Source: CAD feature listing. Evaluate the final solid. Frame: model axes, mm. A direction names the side the tool comes from. Round coordinates to 2 decimals unless told otherwise and drop trailing zeros. Write each loop counter-clockwise with the first axis right and the second up, starting at its lowest first coordinate (ties: lowest second). Pieces come first, ordered by that corner, then holes.
```python
from build123d import *

# Parameters (mm, degrees)
SKETCH1_R           = 2.54
BOSS_EXTRUDE1_DEPTH = 4.699
BOSS_EXTRUDE2_DEPTH = 50.419
FILLET1_R           = 3.81
FILLET2_R           = 2.54
FILLET3_R           = 1.27
SKETCH3_R           = 19.05
BOSS_EXTRUDE3_DEPTH = 1.524
CUT_EXTRUDE1_START  = -6.35
SKETCH5_R           = 22.225
CUT_EXTRUDE1_DEPTH  = 44.45
SKETCH4_R           = 3.175
BOSS_EXTRUDE4_DEPTH = 19.05


with BuildPart() as part:
    # Sketch1 → Boss-Extrude1 (new body)
    with BuildSketch(Plane(origin=(0, 0, 0), x_dir=(1, 0, 0), z_dir=(0, 1, 0))):
        with BuildLine():
            Line((-23.622, 28.575), (23.622, 28.575))
            ThreePointArc((23.622, 28.575), (27.124299887, 27.124299887), (28.575, 23.622))
            Line((28.575, 23.622), (28.575, -23.622))
            ThreePointArc((28.575, -23.622), (27.124299887, -27.124299887), (23.622, -28.575))
            Line((23.622, -28.575), (-23.622, -28.575))
            ThreePointArc((-23.622, -28.575), (-27.124299887, -27.124299887), (-28.575, -23.622))
            Line((-28.575, -23.622), (-28.575, 23.622))
            ThreePointArc((-28.575, 23.622), (-27.124299887, 27.124299887), (-23.622, 28.575))
        make_face()
        with Locations(Location((-23.622, 23.622, 0), (0, 0, 270))):
            Circle(SKETCH1_R, mode=Mode.SUBTRACT)
        with Locations(Location((23.622, 23.622, 0), (0, 0, 270))):
            Circle(SKETCH1_R, mode=Mode.SUBTRACT)
        with Locations(Location((23.622, -23.622, 0), (0, 0, 270))):
            Circle(SKETCH1_R, mode=Mode.SUBTRACT)
        with Locations(Location((-23.622, -23.622, 0), (0, 0, 270))):
            Circle(SKETCH1_R, mode=Mode.SUBTRACT)
    extrude(amount=BOSS_EXTRUDE1_DEPTH)

    # Sketch2 → Boss-Extrude2 (add)
    with BuildSketch(Plane(origin=(0, 4.699, 0), x_dir=(1, 0, 0), z_dir=(0, 1, 0))):
        Polygon((-19.05, -28.575), (-19.05, -19.05), (-28.575, -19.05), (-28.575, 19.05), (-19.05, 19.05), (-19.05, 28.575), (19.05, 28.575), (19.05, 19.05), (28.575, 19.05), (28.575, -19.05), (19.05, -19.05), (19.05, -28.575), align=None)
    extrude(amount=BOSS_EXTRUDE2_DEPTH)

    # Fillet1
    fillet1_edges = [part.edges().sort_by_distance(p)[0] for p in [
        (-19.05, 29.9085, 19.05),
        (-19.05, 29.9085, -19.05),
        (19.05, 29.9085, -19.05),
        (19.05, 29.9085, 19.05),
    ]]
    fillet(fillet1_edges, radius=FILLET1_R)

    # Fillet2
    fillet2_edges = [part.edges().sort_by_distance(p)[0] for p in [
        (28.575, 29.9085, -19.05),
        (19.05, 29.9085, -28.575),
        (28.575, 29.9085, 19.05),
        (-19.05, 29.9085, -28.575),
        (-28.575, 29.9085, -19.05),
        (-19.05, 29.9085, 28.575),
        (-28.575, 29.9085, 19.05),
        (19.05, 29.9085, 28.575),
    ]]
    fillet(fillet2_edges, radius=FILLET2_R)

    # Fillet3
    fillet3_edges = [part.edges().sort_by_distance(p)[0] for p in [
        (24.4475, 55.118, -19.05),
        (28.575, 55.118, 0),
        (0, 55.118, 28.575),
        (19.05, 55.118, 24.4475),
        (0, 55.118, -28.575),
        (-19.05, 55.118, -24.4475),
        (-28.575, 55.118, 0),
        (-24.4475, 55.118, 19.05),
        (18.306051224, 55.118, 27.831051224),
        (-27.831051224, 55.118, 18.306051224),
        (-18.306051224, 55.118, 27.831051224),
        (-27.831051224, 55.118, -18.306051224),
        (-18.306051224, 55.118, -27.831051224),
        (27.831051224, 55.118, 18.306051224),
        (18.306051224, 55.118, -27.831051224),
        (27.831051224, 55.118, -18.306051224),
        (-19.05, 55.118, 24.4475),
        (-24.4475, 55.118, -19.05),
        (19.05, 55.118, -24.4475),
        (24.4475, 55.118, 19.05),
        (-20.165923164, 55.118, 20.165923164),
        (-20.165923164, 55.118, -20.165923164),
        (20.165923164, 55.118, -20.165923164),
        (20.165923164, 55.118, 20.165923164),
    ]]
    fillet(fillet3_edges, radius=FILLET3_R)

    # Sketch3 → Boss-Extrude3 (add)
    with BuildSketch(Plane.XZ):
        with Locations(Location((0, 0, 0), (0, 0, 90))):
            Circle(SKETCH3_R)
    extrude(amount=BOSS_EXTRUDE3_DEPTH)

    # Sketch5 → Cut-Extrude1 (cut)
    with BuildSketch(Plane.XZ.offset(CUT_EXTRUDE1_START)):
        with Locations(Location((0, 0, 0), (0, 0, 270))):
            Circle(SKETCH5_R)
    extrude(amount=-CUT_EXTRUDE1_DEPTH, mode=Mode.SUBTRACT)

    # Sketch4 → Boss-Extrude4 (add)
    with BuildSketch(Plane.XZ.offset(1.524)):
        with Locations(Location((0, 0, 0), (0, 0, 90))):
            Circle(SKETCH4_R)
    extrude(amount=BOSS_EXTRUDE4_DEPTH)


solid = part.part
```
Q1. Section query A-A, the plane y = 16. Output: boundary loops of the cut face in (x, z) (3 decimals), and give its area (3 significant figures).
Q2. Line query: line 1 (Y direction, x = -5, z = -13); line 2 (X direction, y = 25, z = -1) (1 decimal); line 3 (X direction, y = 26, z = 16) (3 decimals). Output: solid intervals per line, ascending.
Q3. Set-up query: faces 5 (the face through (18.286, 29.618, 27.851)), 6 (the face through (-24, 29, -19.05)), 7 (the face through (0, 50.8, 0)), 8 (the face through (27.851, 29.618, -18.286)), 9 (the face through (-21, 4.699, 22)). Return all of +Z, -Z, +X, -X, +Y, -Y with unobstructed straight access to the full face (end or side cutting, diameter ignored); none if empty.
Q4. Section query B-B, the plane x = 0. Output: boundary loops of the cut face in (y, z) (3 decimals).
Q5. Mould query, pull axis Z, two halves, no side actions, for faces 1 (the face through (24.385, 2.317, 26.045)), 2 (the face through (0.4, 0, -19.5)), 3 (the face through (-24.59, 2.32, 25.97)), 4 (the face through (18.286, 29.618, -27.851)). Classes: pulls with the +Z half, pulls with the -Z half, needs draft (parallel to the pull), parting line crosses it, or undercut.
Q6. Pin query (flat end, axial travel): P1, Ø1.6, axis at x = 24.5, y = 26, coming from the -Z side; P2, Ø3.5, axis at x = 25, y = 41, coming from the +Z side; P3, Ø12, axis at x = 7.5, z = -16.5, coming from the -Y side; P4, Ø3, axis at x = 23.622, z = -23.622, coming from the -Y side. Return the tip coordinate at first contact, or that it passes through.
Q7. Section query D-D, the plane y = -3.5. Output: boundary loops of the cut face in (x, z) (3 decimals), and give its area (3 significant figures).
Q8. Section query C-C, the plane z = 0. Output: boundary loops of the cut face in (x, y) (3 decimals).
Filled in:
1. outline: (-28.575, -16.51) arc R2.54 ccw to (-26.035, -19.05) - (-22.86, -19.05) arc R3.81 cw to (-19.05, -22.86) - (-19.05, -26.035) arc R2.54 ccw to (-16.51, -28.575) - (16.51, -28.575) arc R2.54 ccw to (19.05, -26.035) - (19.05, -22.86) arc R3.81 cw to (22.86, -19.05) - (26.035, -19.05) arc R2.54 ccw to (28.575, -16.51) - (28.575, 16.51) arc R2.54 ccw to (26.035, 19.05) - (22.86, 19.05) arc R3.81 cw to (19.05, 22.86) - (19.05, 26.035) arc R2.54 ccw to (16.51, 28.575) - (-16.51, 28.575) arc R2.54 ccw to (-19.05, 26.035) - (-19.05, 22.86) arc R3.81 cw to (-22.86, 19.05) - (-26.035, 19.05) arc R2.54 ccw to (-28.575, 16.51) - close; hole circle Ø44.45 at (0, 0)
1. area: 1,350 mm2
2. line 1: y = -1.52 to 6.35, 50.8 to 55.12
2. line 2: x = -28.6 to -22.2, 22.2 to 28.6
2. line 3: x = -28.575 to -15.426, 15.426 to 28.575
3. face 5: +Z, +X, +Y
3. face 6: -Z, -X, +Y
3. face 7: none
3. face 8: -Z, +X, +Y
3. face 9: +Z, -X, +Y
4. outline: (-20.574, -3.175) - (-1.524, -3.175) - (-1.524, -19.05) - (0, -19.05) - (0, -28.575) - (53.848, -28.575) arc R1.27 ccw to (55.118, -27.305) - (55.118, 27.305) arc R1.27 ccw to (53.848, 28.575) - (0, 28.575) - (0, 19.05) - (-1.524, 19.05) - (-1.524, 3.175) - (-20.574, 3.175) - close; hole (6.35, -22.225) - (50.8, -22.225) - (50.8, 22.225) - (6.35, 22.225) - close
5. face 1: undercut
5. face 2: needs draft
5. face 3: undercut
5. face 4: pulls with the -Z half
6. P1: stops at z = -19.05
6. P2: stops at z = 19.05
6. P3: stops at y = -1.52
6. P4: passes through
7. outline: circle Ø6.35 at (0, 0)
7. area: 31.7 mm2
8. outline: (-28.575, 0) - (-19.05, 0) - (-19.05, -1.524) - (-3.175, -1.524) - (-3.175, -20.574) - (3.175, -20.574) - (3.175, -1.524) - (19.05, -1.524) - (19.05, 0) - (28.575, 0) - (28.575, 53.848) arc R1.27 ccw to (27.305, 55.118) - (-27.305, 55.118) arc R1.27 ccw to (-28.575, 53.848) - close; hole (-22.225, 6.35) - (22.225, 6.35) - (22.225, 50.8) - (-22.225, 50.8) - close
